Design review of the part built by this model. Coordinates are the model's own, in mm. Face numbers are marked on the shaded views. A direction names the side the tool comes from. Coordinates: 2 decimals unless noted, no trailing zeros. Order: outer loops, then holes, each group sorted by start corner. A loop starts at its lowest first (then second) coordinate and runs counter-clockwise, first axis right, second up. Notation, with made-up numbers: (-38.5, 19.5) - (17.5, 19.5) arc R7 cw to (17.5, 25.5) - close; hole circle Ø7 at (18.25, 26.5). An arc over 180 degrees is marked (long way). Write each question's results on one line, items separated by ' | '. Start each with the question number.
```python
from build123d import *

# Parameters (mm, degrees)
SKETCH1_W           = 108
SKETCH1_H           = 73
BOSS_EXTRUDE1_DEPTH = 22
FILLET1_R           = 2
SHELL1_START        = -52
SHELL1_OUTLINE_W    = 20
SHELL1_OUTLINE_H    = 69
SHELL1_DEPTH        = 104
SKETCH6_OUTSIDE_W   = 136.44
SKETCH6_OUTSIDE_H   = 101.44
CUT_EXTRUDE5_DEPTH  = 4


# Read off the part's stored shape, not the designer's step: Shell1
with BuildPart() as part:
    # Sketch1 → Boss-Extrude1 (new body)
    with BuildSketch(Plane(origin=(0, 0, 0), x_dir=(1, 0, 0), z_dir=(0, 1, 0))):
        Rectangle(SKETCH1_W, SKETCH1_H)
    extrude(amount=BOSS_EXTRUDE1_DEPTH)

    # Fillet1
    fillet1_edges = [part.edges().sort_by_distance(p)[0] for p in [
        (54, 11, 36.5),
        (-54, 11, 36.5),
        (-54, 11, -36.5),
        (54, 11, -36.5),
    ]]
    fillet(fillet1_edges, radius=FILLET1_R)

    # Shell1 outline → Shell1 (cut)
    with BuildSketch(Plane.YZ.offset(SHELL1_START)):
        with Locations((12, 0)):
            Rectangle(SHELL1_OUTLINE_W, SHELL1_OUTLINE_H)
    extrude(amount=SHELL1_DEPTH, mode=Mode.SUBTRACT)

    # Sketch6 outside → Cut-Extrude5 (cut)
    with BuildSketch(Plane(origin=(0, 22, 0), x_dir=(1, 0, 0), z_dir=(0, 1, 0))):
        Rectangle(SKETCH6_OUTSIDE_W, SKETCH6_OUTSIDE_H)
        with BuildLine():
            Line((53, -34.5), (53, 34.5))
            ThreePointArc((53, 34.5), (52.707106781, 35.207106781), (52, 35.5))
            Line((52, 35.5), (-52, 35.5))
            ThreePointArc((-52, 35.5), (-52.707106781, 35.207106781), (-53, 34.5))
            Line((-53, 34.5), (-53, -34.5))
            ThreePointArc((-53, -34.5), (-52.707106781, -35.207106781), (-52, -35.5))
            Line((-52, -35.5), (52, -35.5))
            ThreePointArc((52, -35.5), (52.707106781, -35.207106781), (53, -34.5))
        make_face(mode=Mode.SUBTRACT)
    extrude(amount=-CUT_EXTRUDE5_DEPTH, mode=Mode.SUBTRACT)


solid = part.part
```
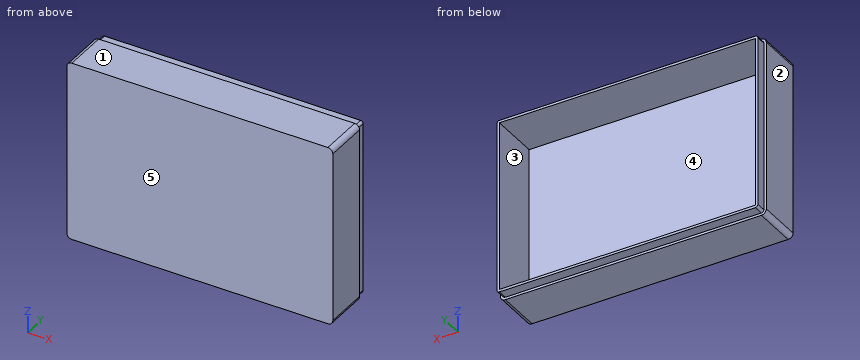
(1) Take a section at C-C (x = 24.5). State the section outline as (y, z) points.
(2) Tool access review of the marked faces 4 and 5: name each direction out of +Z, -Z, +X, -X, +Y, -Y from which nothing blocks a thin tool from reaching the whole face with its end or side.
(3) To check wall thickness, follow line 1 along Z through (x, y) = (41, 9.5); line 2 along X through (y, z) = (15.5, -17); line 3 along X through (y, z) = (20.75, 24). State the ranges of each line that lie inside material, in increasing order. Write a range as [from, to].
(4) Take a section at B-B (z = -1). State the section outline as (x, y) points.
(5) Clearance check with flat-ended pins moving along their axes: pin 1 (3 mm diameter, centred on x = -26, y = 20.5, fed in from +Z); pin 2 (22 mm diameter, centred on x = 26, z = 16, fed in from +Y); pin 3 (1.2 mm diameter, centred on x = 5, y = 20.5, fed in from -Z). State where each tip first meets the part, or that it passes through.
(6) Mouldability with a two-part tool opening along Z and no side actions: class the marked faces 1, 2 and 3 as +Z half, -Z half, draft (parallel to the pull), parting line (faces both ways), or undercut.
(7) Take a section at A-A (y = 14). State the section outline as (x, z) points.
Worked out:
1) outline: (0, -36.5) - (18, -36.5) - (18, -35.5) - (22, -35.5) - (22, -34.5) - (2, -34.5) - (2, 34.5) - (22, 34.5) - (22, 35.5) - (18, 35.5) - (18, 36.5) - (0, 36.5) - close
2) face 4: +Y | face 5: +Z, -Z, +X, -X, -Y
3) line 1: [-36.5, -34.5], [34.5, 36.5] | line 2: [-54, -52], [52, 54] | line 3: [-53, -52], [52, 53]
4) outline: (-54, 0) - (54, 0) - (54, 18) - (53, 18) - (53, 22) - (52, 22) - (52, 2) - (-52, 2) - (-52, 22) - (-53, 22) - (-53, 18) - (-54, 18) - close
5) pin 1: z = 35.5 | pin 2: y = 2 | pin 3: z = -35.5
6) face 1: +Z half | face 2: draft | face 3: undercut
7) outline: (-54, -34.5) arc R2 ccw to (-52, -36.5) - (52, -36.5) arc R2 ccw to (54, -34.5) - (54, 34.5) arc R2 ccw to (52, 36.5) - (-52, 36.5) arc R2 ccw to (-54, 34.5) - close; hole (-52, -34.5) - (52, -34.5) - (52, 34.5) - (-52, 34.5) - close
